from build123d import *

# Parameters (mm, degrees)
F1_DEPTH = 10
F2_R     = 6
F3_DEPTH = 10.001
F4_SIZE  = 0.5


with BuildPart() as f1:
    # F0 (on Right) → F1 (new body)
    with BuildSketch(Plane.YZ):
        Polygon((0, -10.969655), (9.5, -5.484828), (9.5, 5.484828), (0, 10.969655), (-9.5, 5.484828), (-9.5, -5.484828), align=None)
    extrude(amount=-F1_DEPTH)

    # F2 (on face) → F3 (cut, through all)
    with BuildSketch(Plane.YZ):
        Circle(F2_R)
    extrude(amount=-F3_DEPTH, mode=Mode.SUBTRACT)

    # F4
    f4_edges = [f1.edges().sort_by_distance(p)[0] for p in [
        (0, -6, 0),
        (-5, 6, 0),
        (-10, -6, 0),
    ]]
    chamfer(f4_edges, length=F4_SIZE)


solid = f1.part
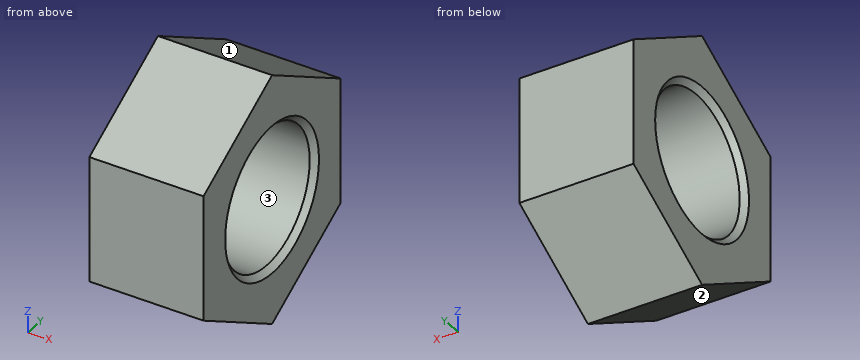
Can you work these out from the model? Positions are in its coordinate system, mm. Face numbers are marked on the shaded views. Round coordinates to 2 decimals unless told otherwise and drop trailing zeros. Loops run counter-clockwise (first coordinate to the right, second up) from the corner with the lowest first, then second, coordinate; pieces in that order, holes last. Notation, with made-up numbers: (86.5, 36) - (98.5, 36) arc R36 ccw to (98.5, 70) - close; hole circle Ø2 at (29.5, 36). An arc over 180 degrees is marked (long way). Answer in a Markdown table with one row per item. Add a question column.
Q1. I need wall thicknesses on L1, parallel to Y at x = -0.25, z = -2.25; L2, parallel to Y at x = -1.5, z = -5.5; L3, parallel to Z at x = -1, y = 4. Which ranges of each line are inside material? Lowest first, please.
Q2. We'd pull the mould along Y, two halves only. Please class the marked faces 1, 2 and 3: pulls with the +Y half, pulls with the -Y half, needs draft (parallel to the pull), parting line crosses it, or undercut.
Q3. For pin 1 Ø5 at (y, z) = (4, 8.5) entering from +X; pin 2 Ø5 at (x, y) = (-3.5, -6.5) entering from -Z; pin 3 Ø4 at (x, y) = (-3, -2.5) entering from +Z, each with a flat end and sliding along its axis, tell me the tip position at first contact or that it passes through.
Q4. I want a section at B-B on x = -2.25. List the corners of the cut face in (y, z) for me.
Q5. I want a section at A-A on z = 0. List the corners of the cut face in (x, y) for me, and give its area (3 significant figures).
Q6. I want a section at C-C on y = 7. List the corners of the cut face in (x, z) for me, and give its area (3 significant figures).
A:
| question | item | result |
|---|---|---|
| 1 | L1 | -9.5 to -5.83, 5.83 to 9.5 |
| 1 | L2 | -9.47 to -2.4, 2.4 to 9.47 |
| 1 | L3 | -8.66 to -4.47, 4.47 to 8.66 |
| 2 | face 1 | pulls with the +Y half |
| 2 | face 2 | pulls with the -Y half |
| 2 | face 3 | undercut |
| 3 | pin 1 | x = 0 |
| 3 | pin 2 | z = -8.66 |
| 3 | pin 3 | z = 10.68 |
| 4 | outline | (-9.5, -5.48) - (0, -10.97) - (9.5, -5.48) - (9.5, 5.48) - (0, 10.97) - (-9.5, 5.48) - close; hole circle Ø12 at (0, 0) |
| 5 | outline | (-10, -9.5) - (0, -9.5) - (0, -6.5) - (-0.5, -6) - (-9.5, -6) - (-10, -6.5) - close; (-10, 6.5) - (-9.5, 6) - (-0.5, 6) - (0, 6.5) - (0, 9.5) - (-10, 9.5) - close |
| 5 | area | 69.5 mm^2 |
| 6 | outline | (-10, -6.93) - (0, -6.93) - (0, 6.93) - (-10, 6.93) - close |
| 6 | area | 139 mm^2 |
